Could you check a few things on this model? Use its own coordinates, in mm. A direction names the side the tool comes from. Give positions to 0.01 mm unless a question says otherwise; leave off trailing zeros. Loops run counter-clockwise (first coordinate to the right, second up) from the corner with the lowest first, then second, coordinate; pieces in that order, holes last. Notation, with made-up numbers: (61, 6) - (107, 6) arc R16 cw to (107, 19) - close; hole circle Ø9 at (36, -34.5). An arc over 180 degrees is marked (long way). One line per item, written item: value. Start each with the question number.
Q1. For faces 1 (the face through (44, 10, 21.25)), 2 (the face through (46, 16.25, 15)), 3 (the face through (29, 10, -26)), 4 (the face through (47.52, 9.94, 9.55)), which set-ups out of +Z, -Z, +X, -X, +Y, -Y let a thin tool reach every point of the face, with its end or its side?
Q2. I want a section at D-D (z = 15.5). Please give me the cut outline in (x, y), then the cut area to 3 significant figures.
Q3. I want a section at C-C (z = -8.5). Please give me the cut outline in (x, y), then the cut area to 3 significant figures.
Q4. I want a section at A-A (x = 42.5). Please give me the cut outline in (y, z), then the cut area to 3 significant figures.
Q5. If I drill on line 1 (Z direction, x = 43, y = 13.5); line 2 (Z direction, x = 29.5, y = 11.5); line 3 (Y direction, x = 12.75, z = -25.35), over which ranges is the centre line in solid material (lowest first)? Write a range as from..to.
Q6. I'm going to push flat-ended pins straight in: P1, Ø1.2, axis at y = 10, z = 19, coming from the +X side; P2, Ø2, axis at y = 9, z = 18, coming from the -X side; P3, Ø2.5, axis at x = 43.5, y = 9, coming from the -Z side; P4, Ø1, axis at y = 2.5, z = -1, coming from the -X side. Where does each tip first touch, or does it pass through?
Q7. I want a section at B-B (x = 12.75). Please give me the cut outline in (y, z).
Q8. If we mould it in two halves opening along X, with no side actions, what happens to faces 5 (the face through (21.14, 12.515, -26.24)), 6 (the face through (45.55, 15, -5)), 7 (the face through (46, 3.75, 15))? For each: released by +X, released by -X, zero draft, split by the parting line, or undercut.
Autodesk Inventor part; units mm, degrees
ref_plane "YZ Plane" through (0, 0, 0) normal (1, 0, 0) x (0, 1, 0)
ref_plane "XZ Plane" through (0, 0, 0) normal (0, 1, 0) x (-1, 0, 0)
ref_plane "XY Plane" through (0, 0, 0) normal (0, 0, 1) x (1, 0, 0)
sketch "スケッチ1" plane through (0, 0, 0) normal (0, 1, 0) x (-1, 0, 0)
  line L0 (0, 40.53276) -> (0, -53.904718)
  line L1 (35.916481, 0) -> (-80.691414, 0)
  line L2 (0, -24.4) -> (-49.55, -24.4)
  line L3 (-49.55, -24.4) -> (-49.55, 24.4)
  line L4 (-49.55, 24.4) -> (0, 24.4)
  line L5 (0, 24.4) -> (0, 22)
  line L6 (0, 22) -> (-46.75, 22)
  line L7 (-46.75, 22) -> (-46.75, -22)
  line L8 (-46.75, -22) -> (0, -22)
  line L9 (0, -24.4) -> (0, -22)
  line L10 (-12.75, -24.4) -> (-12.75, 24.4)
  point P0 (0, 0)
  dimension "d0" = 44
  dimension "d1" = 2.4
  dimension "d2" = 12.75
  dimension "d3" = 34
  dimension "d4" = 2.8
  dimension "d5" = 2.4
sketch "スケッチ1 outline for 押し出し1" plane through (0, 0, 0) normal (0, 1, 0) x (-1, 0, 0)
  line L0 (0, -22) -> (-46.75, -22)
  line L1 (0, -24.4) -> (0, -22)
  line L2 (-49.55, -24.4) -> (0, -24.4)
  line L3 (-49.55, 24.4) -> (-49.55, -24.4)
  line L4 (0, 24.4) -> (-49.55, 24.4)
  line L5 (0, 22) -> (0, 24.4)
  line L6 (-46.75, 22) -> (0, 22)
  line L7 (-46.75, -22) -> (-46.75, 22)
extrude "押し出し1" add sketch "スケッチ1 outline for 押し出し1" along normal blind 20
sketch "スケッチ2" plane through (49.55, 0, -24.4) normal (0, 0, -1) x (-1, 0, 0)
  line L0 (49.55, 20) -> (2.8, 20)
  line L1 (36.8, 20) -> (36.8, 0)
  line L2 (0, 0) -> (49.55, 0)
  line L3 (49.55, 0) -> (49.55, 20)
  line L4 (49.55, 10) -> (0, 10)
  line L5 (0, 0) -> (0, 20)
  circle A0 centre (36.8, 10) radius 3.75
  arc A1 (22.438626, 12.043639) -> (22.438626, 7.956361) centre (22.6, 10) ccw
  line L6 (34.55, 13) -> (22.438626, 12.043639)
  line L7 (34.55, 7) -> (22.438626, 7.956361)
  circle A2 centre (24.3, 10) radius 1
  circle A3 centre (36.8, 10) radius 5.75
  line L8 (33.879857, 14.953309) -> (22.281189, 14.037432)
  arc A4 (22.281189, 14.037432) -> (22.281189, 5.962568) centre (22.6, 10) ccw
  line L9 (22.281189, 5.962568) -> (33.879857, 5.046691)
  dimension "d9" = 7.5
  dimension "d8" = 12.75
  dimension "d10" = 2.05
  dimension "d11" = 14.2
  dimension "d12" = 12.5
  dimension "d13" = 2
  dimension "d14" = 6
  dimension "d43" = 2
  dimension "d44" = 2
sketch "スケッチ2 outline for 押し出し2" plane through (49.55, 0, -24.4) normal (0, 0, -1) x (-1, 0, 0)
  circle A0 centre (36.8, 10) radius 3.75
  circle A1 centre (24.3, 10) radius 1
extrude "押し出し2" cut sketch "スケッチ2 outline for 押し出し2" against normal up to surface (2.4 mm away)
sketch "スケッチ2 outline for 押し出し7" plane through (49.55, 0, -24.4) normal (0, 0, -1) x (-1, 0, 0)
  arc A0 (33.879857, 5.046691) -> (33.879857, 14.953309) centre (36.8, 10) ccw
  line L0 (22.281189, 5.962568) -> (33.879857, 5.046691)
  line L1 (33.879857, 14.953309) -> (22.281189, 14.037432)
  arc A1 (22.281189, 14.037432) -> (22.281189, 5.962568) centre (22.6, 10) ccw
  arc A2 (34.55, 13) -> (34.55, 7) centre (36.8, 10) cw
  line L2 (22.438626, 12.043639) -> (34.55, 13)
  arc A3 (22.438626, 7.956361) -> (22.438626, 12.043639) centre (22.6, 10) cw
  line L3 (34.55, 7) -> (22.438626, 7.956361)
extrude "押し出し7" add sketch "スケッチ2 outline for 押し出し7" along normal blind 2.6
sketch "スケッチ2 outline for 押し出し3" plane through (49.55, 0, -24.4) normal (0, 0, -1) x (-1, 0, 0)
  arc A0 (34.55, 7) -> (34.55, 13) centre (36.8, 10) cw
  line L0 (22.438626, 7.956361) -> (34.55, 7)
  line L1 (34.55, 13) -> (22.438626, 12.043639)
  arc A1 (22.438626, 12.043639) -> (22.438626, 7.956361) centre (22.6, 10) ccw
  circle A2 centre (24.3, 10) radius 1
extrude "押し出し3" add sketch "スケッチ2 outline for 押し出し3" along normal blind 1.1
sketch "スケッチ3" plane through (0, 0, 24.4) normal (0, 0, 1) x (1, 0, 0)
  circle A0 centre (12.75, 10) radius 3.75
  circle A1 centre (12.75, 10) radius 1.75
  point P0 (0, 0)
  dimension "d19" = 3.5
sketch "スケッチ3 outline for 押し出し4" plane through (0, 0, 24.4) normal (0, 0, 1) x (1, 0, 0)
  circle A0 centre (12.75, 10) radius 1.75
extrude "押し出し4" cut sketch "スケッチ3 outline for 押し出し4" against normal up to surface (2.4 mm away)
sketch "スケッチ4" plane through (46.75, 0, -22) normal (-1, 0, 0) x (0, 0, 1)
  line L0 (22, 0) -> (22, 20)
  line L1 (0, 0) -> (0, 20)
  line L2 (0, 10) -> (44, 10)
  line L3 (44, 0) -> (44, 20)
  line L4 (43.25, 16.25) -> (11.25, 16.25)
  line L5 (11.25, 16.25) -> (11.25, 3.75)
  line L6 (11.25, 3.75) -> (43.25, 3.75)
  line L7 (43.25, 3.75) -> (43.25, 16.25)
  line L8 (15.75, 16.25) -> (15.75, 3.75)
  line L9 (38.75, 16.25) -> (38.75, 3.75)
  circle A0 centre (13.5, 10) radius 1
  circle A1 centre (41, 10) radius 1
  arc A2 (27.58771, 12.8) -> (27.58771, 7.2) centre (22, 10) ccw
  arc A3 (28.75, 7.2) -> (28.75, 12.8) centre (28.75, 10) ccw
  line L10 (28.75, 12.8) -> (27.58771, 12.8)
  line L11 (28.75, 7.2) -> (27.58771, 7.2)
  line L12 (15.75, 3.75) -> (15.75, 10)
  point P0 (22, 10)
  point P1 (15.75, 10)
  point P2 (22, 3.75)
  point P3 (22, 16.25)
  dimension "d22" = 4.5
  dimension "d23" = 4.5
  dimension "d24" = 23
  dimension "d25" = 12.5
  dimension "d29" = 2
  dimension "d30" = 2.25
  dimension "d31" = 2.25
  dimension "d39" = 13
  dimension "d40" = 2.8
sketch "スケッチ4 outline for 押し出し5" plane through (46.75, 0, -22) normal (-1, 0, 0) x (0, 0, 1)
  circle A0 centre (41, 10) radius 1
  circle A1 centre (13.5, 10) radius 1
  arc A2 (27.58771, 12.8) -> (27.58771, 7.2) centre (22, 10) ccw
  line L0 (28.75, 12.8) -> (27.58771, 12.8)
  arc A3 (28.75, 7.2) -> (28.75, 12.8) centre (28.75, 10) ccw
  line L1 (27.58771, 7.2) -> (28.75, 7.2)
extrude "押し出し5" cut sketch "スケッチ4 outline for 押し出し5" against normal through all
sketch "スケッチ4 outline for 押し出し8" plane through (46.75, 0, -22) normal (-1, 0, 0) x (0, 0, 1)
  line L0 (15.75, 10) -> (15.75, 3.75)
  arc A0 (22, 3.75) -> (15.75, 10) centre (22, 10) cw
  line L1 (15.75, 3.75) -> (22, 3.75)
  arc A1 (15.75, 10) -> (22, 16.25) centre (22, 10) cw
  line L2 (15.75, 16.25) -> (15.75, 10)
  line L3 (22, 16.25) -> (15.75, 16.25)
  line L4 (28.75, 7.2) -> (27.58771, 7.2)
  arc A2 (28.75, 12.8) -> (28.75, 7.2) centre (28.75, 10) cw
  line L5 (27.58771, 12.8) -> (28.75, 12.8)
  arc A3 (22, 16.25) -> (27.58771, 12.8) centre (22, 10) cw
  line L6 (38.75, 16.25) -> (22, 16.25)
  line L7 (38.75, 3.75) -> (38.75, 16.25)
  line L8 (22, 3.75) -> (38.75, 3.75)
  arc A4 (27.58771, 7.2) -> (22, 3.75) centre (22, 10) cw
extrude "押し出し8" add sketch "スケッチ4 outline for 押し出し8" along normal blind 1.2 contours A0 L1 L0 | L2 L3 A1 | A4 L4 A2 L5 A3 L6 L7 L8
sketch "スケッチ4 outline for 押し出し6" plane through (46.75, 0, -22) normal (-1, 0, 0) x (0, 0, 1)
  line L0 (43.25, 3.75) -> (43.25, 16.25)
  line L1 (38.75, 3.75) -> (43.25, 3.75)
  line L2 (43.25, 16.25) -> (38.75, 16.25)
  line L3 (38.75, 16.25) -> (38.75, 3.75)
  circle A0 centre (41, 10) radius 1
  line L4 (15.75, 3.75) -> (15.75, 16.25)
  line L5 (11.25, 3.75) -> (15.75, 3.75)
  line L6 (15.75, 16.25) -> (11.25, 16.25)
  line L7 (11.25, 16.25) -> (11.25, 3.75)
  circle A1 centre (13.5, 10) radius 1
extrude "押し出し6" add sketch "スケッチ4 outline for 押し出し6" along normal blind 5.2
properties part number "joint3"
Worked answers:
1. face 1: -X, +Y, -Y
1. face 2: -X, +Y
1. face 3: -Z
1. face 4: +X, -X
2. outline: (45.55, 3.75) - (46.75, 3.75) - (46.75, 0) - (49.55, 0) - (49.55, 20) - (46.75, 20) - (46.75, 16.25) - (45.55, 16.25) - close
2. area: 71.0 mm²
3. outline: (41.55, 3.75) - (46.75, 3.75) - (46.75, 0) - (49.55, 0) - (49.55, 9) - (41.55, 9) - close; (41.55, 11) - (49.55, 11) - (49.55, 20) - (46.75, 20) - (46.75, 16.25) - (41.55, 16.25) - close
3. area: 105 mm²
4. outline: (0, -24.4) - (20, -24.4) - (20, -22) - (0, -22) - close; (0, 22) - (20, 22) - (20, 24.4) - (0, 24.4) - close; (3.75, -10.75) - (16.25, -10.75) - (16.25, -6.25) - (3.75, -6.25) - close; (3.75, 16.75) - (16.25, 16.75) - (16.25, 21.25) - (3.75, 21.25) - close; hole circle Ø2 at (10, -8.5); hole circle Ø2 at (10, 19)
4. area: 202 mm²
5. line 1: z = -24.4..-22, -10.75..-6.25, 16.75..21.25, 22..24.4
5. line 2: z = -27..-22, 22..24.4
5. line 3: y = 4.25..6.25, 13.75..15.75
6. P1: passes through
6. P2: stops at x = 41.55
6. P3: stops at z = -24.4
6. P4: stops at x = 46.75
7. outline: (0, -24.4) - (4.25, -24.4) - (4.25, -27) - (6.25, -27) - (6.25, -22) - (0, -22) - close; (0, 22) - (8.25, 22) - (8.25, 24.4) - (0, 24.4) - close; (11.75, 22) - (20, 22) - (20, 24.4) - (11.75, 24.4) - close; (13.75, -27) - (15.75, -27) - (15.75, -24.4) - (20, -24.4) - (20, -22) - (13.75, -22) - close
8. face 5: undercut
8. face 6: released by -X
8. face 7: zero draft
